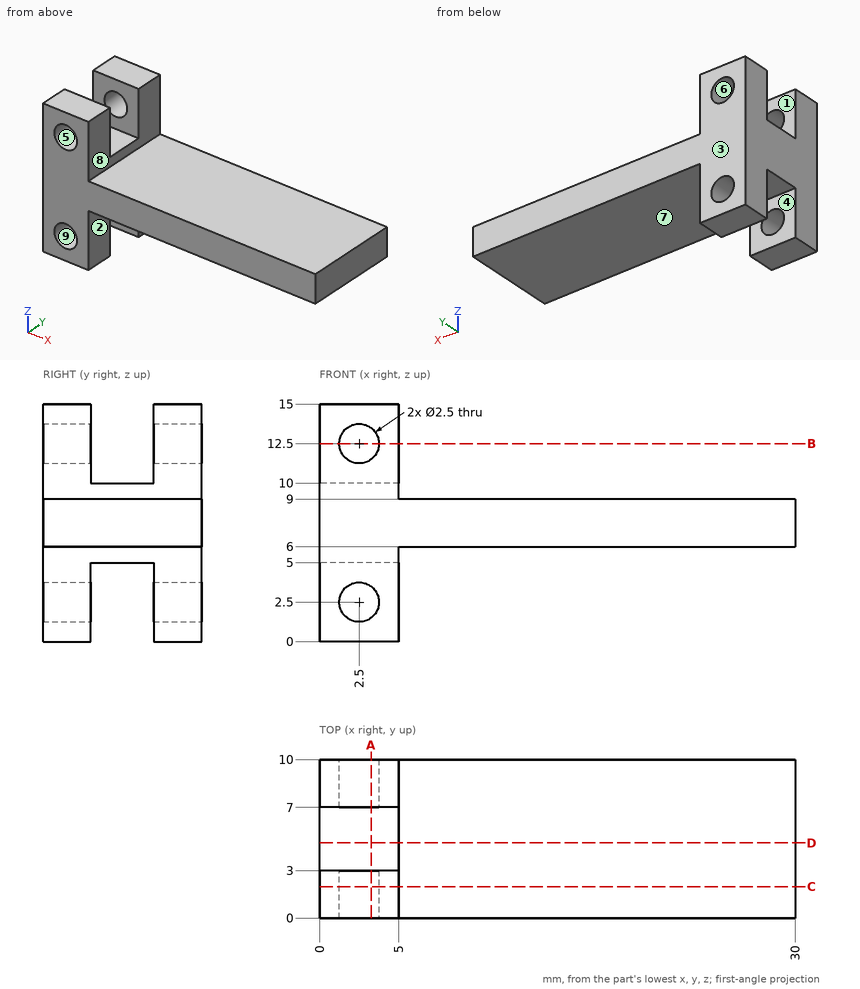
Can you work these out from the drawing? Everything is in mm from the part's minimum corner. A direction names the side the tool comes from. Give positions to 0.01 mm unless a question says otherwise; leave off trailing zeros. Loops run counter-clockwise (first coordinate to the right, second up) from the corner with the lowest first, then second, coordinate; pieces in that order, holes last. Notation, with made-up numbers: (-9, -20.75) -> (30, -20.75) arc R32 cw to (30, 16.25) -> close; hole circle Ø1 at (34.25, 3). An arc over 180 degrees is marked (long way). Return JSON: item names as keys, results as strings.
Q1. I want a section at C-C, the plane y = 2. List the corners of the cut face in (x, z) for me, then the cut area to 3 significant figures.
Checks:
{"outline": "(0, 0) -> (5, 0) -> (5, 6) -> (30, 6) -> (30, 9) -> (5, 9) -> (5, 15) -> (0, 15) -> close; hole circle Ø2.5 at (2.5, 2.5); hole circle Ø2.5 at (2.5, 12.5)", "area": "140 mm2"}
Q2. For pin 1 Ø5 at (x, z) = (23, 12.5) entering from -Y; pin 2 Ø3 at (x, y) = (20, 7) entering from -Z; pin 3 Ø1.8 at (y, z) = (4.5, 4.5) entering from +X; pin 4 Ø5 at (x, y) = (15.5, 3) entering from +Z, each with a flat end and sliding along its axis, tell me the tip position at first contact or that it passes through.
Checks:
{"pin 1": "passes through", "pin 2": "stops at z = 6", "pin 3": "stops at x = 5", "pin 4": "stops at z = 9"}
Q3. On a 3-axis mill with a long thin cutter (end or side, diameter ignored), from which of +Z, -Z, +X, -X, +Y, -Y can I reach the whole of each face in a straight line? I mean the marked faces 1, 2, 3, 4 and 5. Say none if no direction works.
Checks:
{"face 1": "+Z, +X, -X", "face 2": "-Z, +X, +Y, -Y", "face 3": "+Z, -Z, +X, -X, +Y", "face 4": "-Z, +X, -X", "face 5": "+Y, -Y"}
Q4. I want a section at A-A, the plane x = 3.25. List the corners of the cut face in (y, z) for me, then the cut area to 3 significant figures.
Checks:
{"outline": "(0, 0) -> (3, 0) -> (3, 1.5) -> (0, 1.5) -> close; (0, 3.5) -> (3, 3.5) -> (3, 5) -> (7, 5) -> (7, 3.5) -> (10, 3.5) -> (10, 11.5) -> (7, 11.5) -> (7, 10) -> (3, 10) -> (3, 11.5) -> (0, 11.5) -> close; (0, 13.5) -> (3, 13.5) -> (3, 15) -> (0, 15) -> close; (7, 0) -> (10, 0) -> (10, 1.5) -> (7, 1.5) -> close; (7, 13.5) -> (10, 13.5) -> (10, 15) -> (7, 15) -> close", "area": "86.0 mm2"}
Q5. I need wall thicknesses on probe 1 along Z at (x, y) = (2.5, 0.75); probe 2 along X at (y, z) = (2, 2.5); probe 3 along Z at (x, y) = (7.25, 5). Which ranges of each line are inside material? Lowest first, please.
Checks:
{"probe 1": "z = 0 to 1.25, 3.75 to 11.25, 13.75 to 15", "probe 2": "x = 0 to 1.25, 3.75 to 5", "probe 3": "z = 6 to 9"}
Q6. I want a section at D-D, the plane y = 4.75. List the corners of the cut face in (x, z) for me, then the cut area to 3 significant figures.
Checks:
{"outline": "(0, 5) -> (5, 5) -> (5, 6) -> (30, 6) -> (30, 9) -> (5, 9) -> (5, 10) -> (0, 10) -> close", "area": "100 mm2"}
Q7. We'd pull the mould along X, two halves only. Please class the marked faces 6, 7, 8 and 9: released by +X, released by -X, zero draft, split by the parting line, or undercut.
Checks:
{"face 6": "undercut", "face 7": "zero draft", "face 8": "released by +X", "face 9": "undercut"}
Q8. I want a section at B-B, the plane z = 12.5. List the corners of the cut face in (x, y) for me.
Checks:
{"outline": "(0, 0) -> (1.25, 0) -> (1.25, 3) -> (0, 3) -> close; (0, 7) -> (1.25, 7) -> (1.25, 10) -> (0, 10) -> close; (3.75, 0) -> (5, 0) -> (5, 3) -> (3.75, 3) -> close; (3.75, 7) -> (5, 7) -> (5, 10) -> (3.75, 10) -> close"}
